from build123d import *

# Parameters (mm, degrees)
F0_W        = 20.32
F0_H        = 50.8
F1_DEPTH    = 7.62
F2_D        = 6.35
F3_R        = 6.35
F4_D        = 17.78
F5_DEPTH    = 25.4
F6_T1_DEPTH = 138.2614957887
F7_R        = 7.62
F9_DEPTH    = 25.4
F11_D       = 4.318
F11_DEPTH   = 5.08
F11_TIP     = 1.2972580765
F12_D       = 3.556
F13_R       = 9.525
F13_R_2     = 1.778
F14_DEPTH   = 7.62
F10_W       = 5.588
F10_H       = 25.4
F16_DEPTH   = 15.24
F17_DEPTH   = 25.4


# Not quite as in the source:
# - a fillet or chamfer that OpenCascade refuses, or shapes differently, is made with other operations: its cross-section is extruded or revolved along the edge and cut away or added


with BuildPart() as f1:
    # F0 (on Top) → F1 (new body)
    with BuildSketch(Plane.XY):
        Polygon((46.4461110532, 37.6075126914), (-42.4538889468, 37.6075126914), (-42.4538889468, -51.2924873086), (46.4461110532, -51.2924873086), (46.4461110532, -32.2424873086), (26.1261110532, -32.2424873086), (26.1261110532, 18.5575126914), (46.4461110532, 18.5575126914), align=None)
        with Locations((36.2861110532, -6.8424873086)):
            Rectangle(F0_W, F0_H)
    extrude(amount=F1_DEPTH)

    # F2 (through all)
    with Locations(Plane(origin=(0, 0, 0), x_dir=(1, 0, 0), z_dir=(0, 0, -1))):
        with Locations((-32.5478889468, -27.7015126914), (36.5401110532, -27.7015126914), (36.5401110532, 41.3864873086), (-32.5478889468, 41.3864873086)):
            Hole(F2_D / 2)

    # F3
    f3_edges = [f1.edges().sort_by_distance(p)[0] for p in [
        (-42.453889, -51.292487, 3.81),
        (46.446111, -51.292487, 3.81),
        (46.446111, 37.607513, 3.81),
        (-42.453889, 37.607513, 3.81),
    ]]
    fillet(f3_edges, radius=F3_R)

    # F4 (through all)
    with Locations(Plane(origin=(0, 0, 0), x_dir=(1, 0, 0), z_dir=(0, 0, -1))):
        with Locations((1.9961110532, 6.8424873086)):
            Hole(F4_D / 2)

    # F5 (add): a face of the model
    f5_faces = [f1.faces().sort_by_distance(p)[0] for p in [
        (1.9961110532, -51.2924873086, 3.81),
    ]]
    extrude(f5_faces, amount=F5_DEPTH)

    # F6: chamfer of 25.4 on 3 edges, made by hand

    # F6_s2 → F6_t1 (cut)
    with BuildSketch(Plane.XY.offset(-65.3207478943)):
        Polygon((40.0961110532, -51.2924873086), (14.6961110532, -76.6924873086), (40.0961110532, -76.6924873086), align=None)
        Polygon((-36.1038889468, -51.2924873086), (-10.7038889468, -76.6924873086), (-36.1038889468, -76.6924873086), align=None)
    extrude(amount=F6_T1_DEPTH, mode=Mode.SUBTRACT)

    # F7
    f7_edges = [f1.edges().sort_by_distance(p)[0] for p in [
        (14.696111, -76.692487, 3.81),
        (-10.703889, -76.692487, 3.81),
    ]]
    fillet(f7_edges, radius=F7_R)

    # F8 (on face) → F9 (join)
    with BuildSketch(Plane.XY.offset(7.62)):
        with BuildLine():
            Line((24.8561110532, -66.5324873086), (-20.8638889468, -66.5324873086))
            Line((-20.8638889468, -66.5324873086), (-12.9357352742, -74.4606409812))
            ThreePointArc((-12.9357352742, -74.4606409812), (-10.4636293562, -76.1124493463), (-7.5475816015, -76.6924873086))
            Line((-7.5475816015, -76.6924873086), (11.5398037079, -76.6924873086))
            ThreePointArc((11.5398037079, -76.6924873086), (14.4558514626, -76.1124493463), (16.9279573806, -74.4606409812))
            Line((16.9279573806, -74.4606409812), (24.8561110532, -66.5324873086))
        make_face()
    extrude(amount=F9_DEPTH)

    # F11
    with Locations(Plane(origin=(0, -66.5324873086, 0), x_dir=(-1, 0, 0), z_dir=(0, 1, 0))):
        with Locations((-14.6961110532, 22.098), (10.7038889468, 22.098)):
            Hole(F11_D / 2, depth=F11_DEPTH)
            with Locations((0, 0, -(F11_DEPTH + F11_TIP / 2))):  # 118° drill point
                Cone(0, F11_D / 2, F11_TIP, mode=Mode.SUBTRACT)

    # F12 (through all)
    with Locations(Plane(origin=(0, -66.5324873086, 0), x_dir=(-1, 0, 0), z_dir=(0, 1, 0))):
        with Locations((-1.9961110532, 22.098)):
            Hole(F12_D / 2)

    # F13 (on face) → F14 (cut)
    with BuildSketch(Plane.XZ.offset(76.6924873086)):
        with Locations((1.9961110532, 22.098)):
            Circle(F13_R)
        with Locations((1.9961110532, 22.098)):
            Circle(F13_R_2, mode=Mode.SUBTRACT)
    extrude(amount=-F14_DEPTH, mode=Mode.SUBTRACT)

    # F10 (on face) → F16 (join)
    with BuildSketch(Plane(origin=(0, -66.5324873086, 0), x_dir=(-1, 0, 0), z_dir=(0, 1, 0))):
        with Locations((-22.0621110532, 20.32)):
            Rectangle(F10_W, F10_H)
        with Locations((18.0698889468, 20.32)):
            Rectangle(F10_W, F10_H)
    extrude(amount=F16_DEPTH)

    # F15 (on face) → F17 (join)
    with BuildSketch(Plane.XY.offset(7.62)):
        Polygon((24.8561110532, -66.5324873086), (40.0961110532, -51.2924873086), (24.8561110532, -51.2924873086), align=None)
        Polygon((-36.1038889468, -51.2924873086), (-20.8638889468, -66.5324873086), (-20.8638889468, -51.2924873086), align=None)
    extrude(amount=F17_DEPTH)


solid = f1.part
Here's how the part is built. I have some questions about the finished solid (model axes, mm). A direction names the side the tool comes from. Coordinates: 2 decimals unless noted, no trailing zeros. Order: outer loops, then holes, each group sorted by start corner. A loop starts at its lowest first (then second) coordinate and runs counter-clockwise, first axis right, second up. Notation, with made-up numbers: (-2, 46.5) -> (50, 46.5) arc R18 cw to (50, 64.5) -> close; hole circle Ø3 at (-27, 54). An arc over 180 degrees is marked (long way). Answer in a Markdown table with one row per item.
(1) Thinking about a two-plate mould opening in Z: for faces 1 (the face through (-10.406, -72.684, 21.87)), 2 (the face through (3, 37.608, 4)), 3 (the face through (1, -67, 33.02)), which applies, +Z half, -Z half, draft (parallel to the pull), parting line (faces both ways), or undercut?
Answer key:
| item | result |
|---|---|
| face 1 | undercut |
| face 2 | draft |
| face 3 | +Z half |
(2) I want a section at D-D on y = -24. List the corners of the cut face in (x, z) for me, then the cut area to 3 significant figures.
Answer key:
| item | result |
|---|---|
| outline | (-42.45, 0) -> (46.45, 0) -> (46.45, 7.62) -> (-42.45, 7.62) -> close |
| area | 677 mm^2 |
(3) I want a section at A-A on x = 6. List the corners of the cut face in (y, z) for me.
Answer key:
| item | result |
|---|---|
| outline | (-76.69, 0) -> (-14.78, 0) -> (-14.78, 7.62) -> (-66.53, 7.62) -> (-66.53, 33.02) -> (-76.69, 33.02) -> (-76.69, 30.74) -> (-69.07, 30.74) -> (-69.07, 13.46) -> (-76.69, 13.46) -> close; (1.09, 0) -> (37.61, 0) -> (37.61, 7.62) -> (1.09, 7.62) -> close |
(4) On a 3-axis mill with a long thin cutter (end or side, diameter ignored), from which of +Z, -Z, +X, -X, +Y, -Y can I reach the whole of each face in a straight line? I mean faces 4 (the face through (-0.07, -72.94, 12.8)), 5 (the face through (2, -66.532, 20)), 6 (the face through (15.857, -69.108, 23.918)). Say none if no direction works.
Answer key:
| item | result |
|---|---|
| face 4 | -Y |
| face 5 | +Z, +Y |
| face 6 | +Y |
(5) Will these pins go through, and if not, where does the flat tip stop? pin 1 Ø10.5 at (x, z) = (28, 16) entering from +Y; pin 2 Ø15 at (x, z) = (0.5, 20.5) entering from -Y; pin 3 Ø17 at (y, z) = (-62.5, 16) entering from +X; pin 4 Ø8 at (x, y) = (-19.5, -24.5) entering from +Z.
Answer key:
| item | result |
|---|---|
| pin 1 | y = -51.29 |
| pin 2 | y = -76.69 |
| pin 3 | x = 37.39 |
| pin 4 | z = 7.62 |
(6) I want a section at C-C on z = 29.5. List the corners of the cut face in (x, y) for me, then the cut area to 3 significant figures.
Answer key:
| item | result |
|---|---|
| outline | (-36.1, -51.29) -> (-12.94, -74.46) arc R7.62 ccw to (-7.55, -76.69) -> (-4, -76.69) -> (-4, -69.07) -> (7.99, -69.07) -> (7.99, -76.69) -> (11.54, -76.69) arc R7.62 ccw to (16.93, -74.46) -> (40.1, -51.29) -> (19.27, -51.29) -> (19.27, -66.53) -> (-15.28, -66.53) -> (-15.28, -51.29) -> close |
| area | 670 mm^2 |
(7) I want a section at B-B on y = -3.5. List the corners of the cut face in (x, z) for me.
Answer key:
| item | result |
|---|---|
| outline | (-42.45, 0) -> (-6.24, 0) -> (-6.24, 7.62) -> (-42.45, 7.62) -> close; (10.23, 0) -> (46.45, 0) -> (46.45, 7.62) -> (10.23, 7.62) -> close |
(8) Please list where these lines run through material, in increasing order: probe 1 along X at (y, z) = (28.5, 2.5); probe 2 along Z at (x, y) = (2, -46.5); probe 3 along Y at (x, z) = (-3.5, 28.5).
Answer key:
| item | result |
|---|---|
| probe 1 | -42.45 to -35.62, -29.47 to 33.47, 39.61 to 46.45 |
| probe 2 | 0 to 7.62 |
| probe 3 | -69.07 to -66.53 |
